The listing builds one solid part. Answer for the finished solid, in the listing's coordinates (mm). A direction names the side the tool comes from. Round coordinates to 2 decimals unless told otherwise and drop trailing zeros. Write each loop counter-clockwise with the first axis right and the second up, starting at its lowest first coordinate (ties: lowest second). Pieces come first, ordered by that corner, then holes.
from build123d import *

# Parameters (mm, degrees)
EXTRUDE_1_DEPTH     = 71
CUT_EXTRUDE_2_DEPTH = 71
SKETCH_3_W          = 28.502340284
SKETCH_3_H          = 18.562195974
CUT_EXTRUDE_3_DEPTH = 71
EXTRUDE_4_DEPTH     = 3
SKETCH_5_R          = 1.5
CUT_EXTRUDE_5_DEPTH = 10
SKETCH_6_R          = 4.5
CUT_EXTRUDE_6_DEPTH = 10
SKETCH_8_R          = 2.1
CUT_EXTRUDE_7_DEPTH = 15
SKETCH_9_R          = 2.1
CUT_EXTRUDE_8_DEPTH = 101.617881054


with BuildPart() as part:
    # 草图1 → 拉伸1 (new body)
    with BuildSketch(Plane.XY):
        with BuildLine():
            Line((-32.966640689, -19.89344536), (-32.966640689, 39.10655464))
            Line((-32.966640689, 39.10655464), (0.356973729, 39.10655464))
            ThreePointArc((0.356973729, 39.10655464), (1.820381254, 38.725416686), (2.911948679, 37.678846917))
            Line((2.911948679, 37.678846917), (9.588334261, 26.829720346))
            ThreePointArc((9.588334261, 26.829720346), (9.919959807, 26.074457796), (10.033359311, 25.257428069))
            Line((10.033359311, 25.257428069), (10.033359311, 15.782940222))
            ThreePointArc((10.033359311, 15.782940222), (9.652221357, 14.319532697), (8.605651588, 13.227965272))
            Line((8.605651588, 13.227965272), (1.286230543, 8.723706168))
            ThreePointArc((1.286230543, 8.723706168), (0.321919702, 7.770494191), (-0.124217104, 6.490076126))
            Line((-0.124217104, 6.490076126), (-2.966640689, -19.89344536))
            Line((-2.966640689, -19.89344536), (-12.966640689, -19.89344536))
            Line((-12.966640689, -19.89344536), (-12.966640689, -4.89344536))
            ThreePointArc((-12.966640689, -4.89344536), (-17.966640689, 0.10655464), (-22.966640689, -4.89344536))
            Line((-22.966640689, -4.89344536), (-22.966640689, -19.89344536))
            Line((-22.966640689, -19.89344536), (-32.966640689, -19.89344536))
        make_face()
    extrude(amount=EXTRUDE_1_DEPTH)

    # 草图2 → 拉伸2 (cut)
    with BuildSketch(Plane.ZY.offset(32.966640689)):
        with BuildLine():
            Line((11, -19.89344536), (11, -2.89344536))
            ThreePointArc((11, -2.89344536), (11.878679656, -0.772125016), (14, 0.10655464))
            Line((14, 0.10655464), (57, 0.10655464))
            ThreePointArc((57, 0.10655464), (59.121320344, -0.772125016), (60, -2.89344536))
            Line((60, -2.89344536), (60, -19.89344536))
            Line((60, -19.89344536), (11, -19.89344536))
        make_face()
    extrude(amount=-CUT_EXTRUDE_2_DEPTH, mode=Mode.SUBTRACT)

    # 草图3 → 拉伸3 (cut)
    with BuildSketch(Plane.XY.offset(71)):
        with Locations((-14.251170142, 23.589261476)):
            Rectangle(SKETCH_3_W, SKETCH_3_H)
    extrude(amount=-CUT_EXTRUDE_3_DEPTH, mode=Mode.SUBTRACT)

    # 草图4 → 拉伸4 (add)
    with BuildSketch(Plane.XY.offset(71)):
        with BuildLine():
            Line((-32.165931594, 13.697564937), (-32.165931594, 35.556993091))
            Line((-32.165931594, 35.556993091), (0.806390202, 37.022429615))
            Line((0.806390202, 37.022429615), (8.68311152, 24.627279014))
            ThreePointArc((8.68311152, 24.627279014), (9.577922468, 21.550792247), (8.68311152, 18.47430548))
            Line((8.68311152, 18.47430548), (0, 10.907326517))
            Line((0, 10.907326517), (-32.165931594, 10.907326517))
            Line((-32.165931594, 10.907326517), (-32.165931594, 13.697564937))
        make_face()
    extrude_4 = extrude(amount=EXTRUDE_4_DEPTH)

    # 草图5 → 拉伸5 (cut)
    with BuildSketch(Plane.XY.offset(74)):
        with Locations((-28.135981152, 32.259760911)):
            Circle(SKETCH_5_R)
        with Locations((0, 34.091556567)):
            Circle(SKETCH_5_R)
        with Locations((-1.049162635, 13.209086096)):
            Circle(SKETCH_5_R)
        with Locations((-28.135981152, 13.209086096)):
            Circle(SKETCH_5_R)
    cut_extrude_5 = extrude(amount=-CUT_EXTRUDE_5_DEPTH, mode=Mode.SUBTRACT)

    # 镜向2: 拉伸4, 拉伸5 across plane
    add(extrude_4.mirror(Plane(origin=(0, 0, 36), x_dir=(1, 0, 0), z_dir=(0, 0, -1))))
    add(cut_extrude_5.mirror(Plane(origin=(0, 0, 36), x_dir=(1, 0, 0), z_dir=(0, 0, -1))), mode=Mode.SUBTRACT)

    # 草图6 → 拉伸6 (cut)
    with BuildSketch(Plane(origin=(0, 39.10655464, 0), x_dir=(1, 0, 0), z_dir=(0, 1, 0))):
        with Locations(Location((-13.466640689, -36, 0), (0, 0, 180))):
            Circle(SKETCH_6_R)
    extrude(amount=-CUT_EXTRUDE_6_DEPTH, mode=Mode.SUBTRACT)

    # 草图7 → 旋转1 (revolve)
    with BuildSketch(Plane(origin=(0, 0, 36), x_dir=(-1, 0, 0), z_dir=(0, 0, -1))):
        Polygon((17.851883619, 32.870359463), (25.473752014, 32.870359463), (25.473752014, 16.752081431), (13.466640689, 16.752081431), (13.466640689, 57.10655464), (17.851883619, 57.10655464), align=None)
    revolve(axis=Axis((-13.466640689, 60.856315585, 36), (0, -1, 0)))

    # 草图8 → 拉伸7 (cut)
    with BuildSketch(Plane.XZ.offset(19.89344536)):
        with Locations(Location((-27.966640689, 65.5, 0), (0, 0, 270))):
            Circle(SKETCH_8_R)
        with Locations(Location((-7.966640689, 66, 0), (0, 0, 270))):
            Circle(SKETCH_8_R)
        with Locations(Location((-27.966640689, 6, 0), (0, 0, 270))):
            Circle(SKETCH_8_R)
        with Locations(Location((-7.966640689, 6, 0), (0, 0, 270))):
            Circle(SKETCH_8_R)
    extrude(amount=-CUT_EXTRUDE_7_DEPTH, mode=Mode.SUBTRACT)

    # 草图9 → 拉伸8 (cut, through all)
    with BuildSketch(Plane(origin=(0, 0, -2), x_dir=(-1, 0, 0), z_dir=(0, 0, -1))):
        with Locations((1.189151156, 23.791556567)):
            Circle(SKETCH_9_R)
    extrude(amount=-CUT_EXTRUDE_8_DEPTH, mode=Mode.SUBTRACT)


solid = part.part
1. Straight lines are drawn through the part: line 1 along Y through (x, z) = (-23, 53); line 2 along Z through (x, y) = (-3, 19); line 3 along Y through (x, z) = (-10.5, 37). For each, find the intervals that lie inside material, in ascending order.
Geometry says:
line 1: y = 0.11 to 14.31, 32.87 to 39.11
line 2: z = -2 to 1, 30.12 to 41.88, 71 to 74
line 3: y = 0.11 to 14.31, 16.75 to 57.11
2. For a pull along Y with two mould halves and no side action, classify faces 5 (the face through (-10.017, -12.498, 6.455)), 6 (the face through (-1.374, 11.745, 69.07)), 7 (the face through (-7.603, -0.796, 11.855)) as released by +Y, released by -Y, zero draft, split by the parting line, or undercut.
Geometry says:
face 5: zero draft
face 6: undercut
face 7: released by -Y
3. A tool of negligible diameter and unlimited length cuts with its end or side. For faces 1 (the face through (-0.2, 35.58, 2.93)), 2 (the face through (-25.885, -12.498, 6.273)), 3 (the face through (-32.166, 23, -1)), 4 (the face through (-7, -12, 11)), from which of +Z, -Z, +X, -X, +Y, -Y can it reach the whole face along a straight path? Write none if from no direction.
Geometry says:
face 1: -Z
face 2: -Y
face 3: -Z, -X, +Y, -Y
face 4: +X, -X, -Y
4. Section B-B on y = 20 is taken. Determine the outline of the cut face in (x, z).
Geometry says:
outline: (-32.97, 0) - (-32.17, 0) - (-32.17, -2) - (9.36, -2) - (9.36, 0) - (10.03, 0) - (10.03, 71) - (9.36, 71) - (9.36, 74) - (-32.17, 74) - (-32.17, 71) - (-32.97, 71) - close; circle Ø24.01 at (-13.47, 36); hole (-28.5, 1) - (0, 1) - (0, 71) - (-28.5, 71) - close
5. Given pin 1 (2.5 mm diameter, centred on x = -28.14, y = 13.21, fed in from +Z); pin 2 (4 mm diameter, centred on x = -1.19, y = 23.79, fed in from -Z); pin 3 (6 mm diameter, centred on x = -10.5, y = -12, fed in from +Z); pin 4 (1.5 mm diameter, centred on x = -28.5, y = 13.5, fed in from -Z), each flat-ended and moving along its own axis, determine where each tip first touches the part or whether it passes through.
Geometry says:
pin 1: stops at z = 64
pin 2: passes through
pin 3: stops at z = 71
pin 4: stops at z = 8
6. Section C-C on x = -20 is taken. Determine the outline of the cut face in (y, z).
Geometry says:
outline: (-0.33, 0) - (10.91, 0) - (10.91, -2) - (36.1, -2) - (36.1, 0) - (39.11, 0) - (39.11, 71) - (36.1, 71) - (36.1, 74) - (10.91, 74) - (10.91, 71) - (-0.33, 71) - (-0.33, 58.55) arc R3 cw to (0.11, 57) - (0.11, 14) arc R3 cw to (-0.33, 12.45) - close; hole (14.31, 1) - (32.87, 1) - (32.87, 25.93) - (16.75, 25.93) - (16.75, 46.07) - (32.87, 46.07) - (32.87, 71) - (14.31, 71) - close
